Build history of the part. All positions in model axes, mm. Face numbers are marked on the shaded views. Coordinates: 2 decimals unless noted, no trailing zeros. Loops run counter-clockwise (first coordinate to the right, second up) from the corner with the lowest first, then second, coordinate; pieces in that order, holes last.
(1) Slice it at B-B (z = 2.25). Give the number of separate pieces and of enclosed holes in the cut face, and give its area (3 significant figures).
(2) Slice it at A-A (x = 0). Give the cut face in (y, z).
(3) Flat gauge pins, fed straight in: P1, Ø17, axis at x = -25.56, y = -19.7, coming from the -Z side; P2, Ø2.5, axis at x = -2.5, z = 2.5, coming from the -Y side; P3, Ø4, axis at x = -13.5, y = -20.5, coming from the -Z side; P4, Ø3.5, axis at y = -2, z = 2.5, coming from the +X side. Where does each tip first touch, or does it go through?
(4) Wall check: L1, parallel to Y at x = 0, z = 2.25; L2, parallel to Y at x = -4.5, z = 1.5; L3, parallel to Y at x = 13, z = 1.5. Give the ranges that are in metal, low to high.
(5) Two-plate mould, pull along X, no slides. Class the marked faces 1, 2 and 3: pulls with the +X half, pulls with the -X half, needs draft (parallel to the pull), parting line crosses it, or undercut.
from build123d import *

# Parameters (mm, degrees)
F0_R     = 10.75
F1_DEPTH = 6.35


with BuildPart() as f1:
    # F0 (on Top) → F1 (new body)
    with BuildSketch(Plane.XY):
        with BuildLine():
            ThreePointArc((-16.446219, 24.955231), (-18.635535, 6.586639), (-31.317256, -6.880812))
            ThreePointArc((-31.317256, -6.880812), (-31.945446, -7.211903), (-32.581411, -7.527802))
            ThreePointArc((-32.581411, -7.527802), (-35.491262, -29.630309), (-13.388754, -26.720459))
            ThreePointArc((-13.388754, -26.720459), (3.613571, -19.432166), (21.617586, -23.681133))
            ThreePointArc((21.617586, -23.681133), (22.218414, -24.059617), (22.809974, -24.452429))
            ThreePointArc((22.809974, -24.452429), (43.406231, -15.921179), (29.834974, 1.765228))
            ThreePointArc((29.834974, 1.765228), (15.021964, 12.845527), (9.69967, 30.561945))
            ThreePointArc((9.69967, 30.561945), (9.727032, 31.271519), (9.771438, 31.980231))
            ThreePointArc((9.771438, 31.980231), (-7.91497, 45.551489), (-16.446219, 24.955231))
        make_face()
        with Locations((-25.556411, -19.695459)):
            Circle(F0_R, mode=Mode.SUBTRACT)
        Polygon((-8.926963, -8.174784), (-10.426963, -10.772861), (-11.926963, -8.174784), align=None, mode=Mode.SUBTRACT)
        Polygon((-3.643584, -11.543052), (-3.643584, -14.543052), (-6.241661, -13.043052), align=None, mode=Mode.SUBTRACT)
        Polygon((-11.818369, -2.61609), (-14.416445, -4.11609), (-14.416445, -1.11609), align=None, mode=Mode.SUBTRACT)
        Polygon((-11.543052, 3.643584), (-14.543052, 3.643584), (-13.043052, 6.241661), align=None, mode=Mode.SUBTRACT)
        with BuildLine():
            ThreePointArc((-10.42615, -2.618758), (-1.319353, 10.66873), (10.75, 0))
            ThreePointArc((10.75, 0), (1.319353, -10.66873), (-10.42615, -2.618758))
        make_face(mode=Mode.SUBTRACT)
        Polygon((2.61609, -11.818369), (4.11609, -14.416445), (1.11609, -14.416445), align=None, mode=Mode.SUBTRACT)
        Polygon((8.174784, -8.926963), (10.772861, -10.426963), (8.174784, -11.926963), align=None, mode=Mode.SUBTRACT)
        Polygon((11.543052, -3.643584), (14.543052, -3.643584), (13.043052, -6.241661), align=None, mode=Mode.SUBTRACT)
        Polygon((11.818369, 2.61609), (14.416445, 4.11609), (14.416445, 1.11609), align=None, mode=Mode.SUBTRACT)
        with BuildLine():
            ThreePointArc((22.592473, -4.340674), (34.176956, -2.450663), (40.584974, -12.284772))
            ThreePointArc((40.584974, -12.284772), (29.91008, -23.034509), (19.086023, -12.434981))
            ThreePointArc((19.086023, -12.434981), (19.970769, -8.011603), (22.592473, -4.340674))
        make_face(mode=Mode.SUBTRACT)
        Polygon((-8.174784, 8.926963), (-10.772861, 10.426963), (-8.174784, 11.926963), align=None, mode=Mode.SUBTRACT)
        Polygon((-2.61609, 11.818369), (-4.11609, 14.416445), (-1.11609, 14.416445), align=None, mode=Mode.SUBTRACT)
        with BuildLine():
            ThreePointArc((-7.0369, 21.590136), (-10.832583, 40.501224), (6.471438, 31.980231))
            ThreePointArc((6.471438, 31.980231), (5.19515, 26.89975), (1.669339, 23.025625))
            ThreePointArc((1.669339, 23.025625), (-2.52971, 21.37344), (-7.0369, 21.590136))
        make_face(mode=Mode.SUBTRACT)
        Polygon((8.926963, 8.174784), (10.426963, 10.772861), (11.926963, 8.174784), align=None, mode=Mode.SUBTRACT)
        Polygon((3.643584, 11.543052), (3.643584, 14.543052), (6.241661, 13.043052), align=None, mode=Mode.SUBTRACT)
    extrude(amount=F1_DEPTH)


solid = f1.part
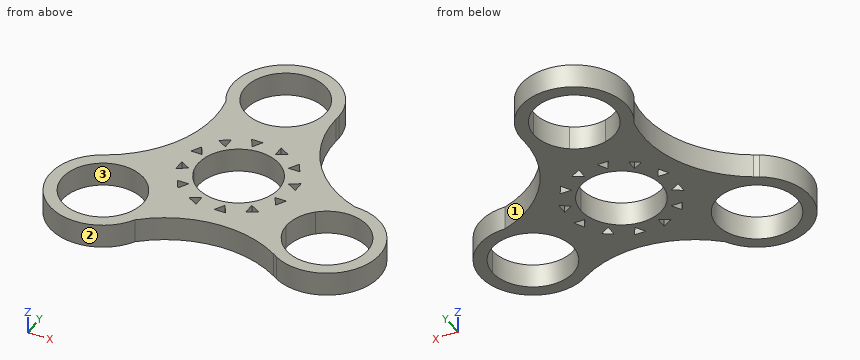
Response values:
1. separate pieces: 1
1. enclosed holes: 16
1. area: 1,830 mm2
2. outline: (-19.97, 0) - (-10.75, 0) - (-10.75, 6.35) - (-19.97, 6.35) - close; (10.75, 0) - (22.12, 0) - (22.12, 6.35) - (10.75, 6.35) - close; (41.84, 0) - (45.36, 0) - (45.36, 6.35) - (41.84, 6.35) - close
3. P1: passes through
3. P2: stops at y = -21.04
3. P3: stops at z = 0
3. P4: stops at x = 41
4. L1: y = -19.97 to -10.75, 10.75 to 22.12, 41.84 to 45.36
4. L2: y = -21.31 to -14.05, -12.04 to -9.76, 9.76 to 21.23, 42.73 to 46.03
4. L3: y = -20.12 to -6.17, -3.64 to 1.93, 3.3 to 16.19
5. face 1: pulls with the +X half
5. face 2: parting line crosses it
5. face 3: undercut
